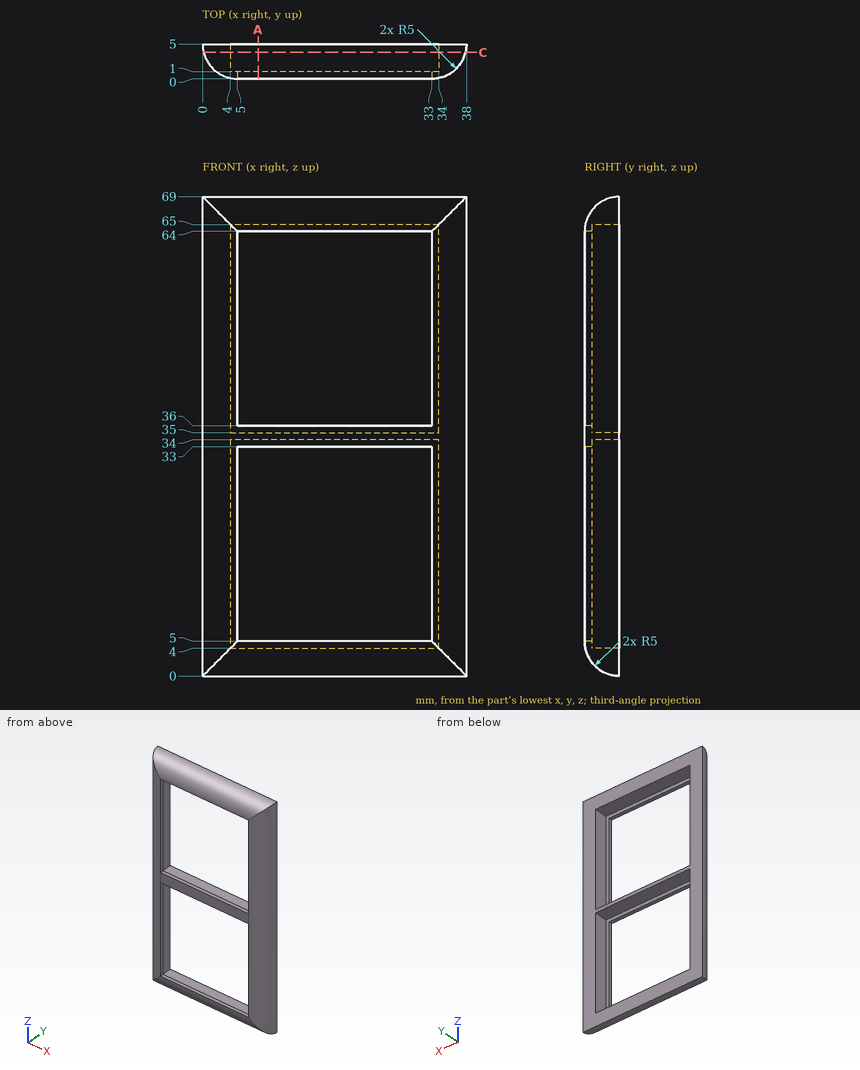
Geometry check sheet. Reference: drawing and pictorial views, mm from the part's lowest x, y, z. Coordinates: 2 decimals unless noted, no trailing zeros. Order: outer loops, then holes, each group sorted by start corner. A loop starts at its lowest first (then second) coordinate and runs counter-clockwise, first axis right, second up.
Item 1: Depth check by flat-ended pin: pin 1 (1.1 mm diameter, centred on y = 0.5, z = 17.5, fed in from -X); pin 2 (1.1 mm diameter, centred on y = 0.5, z = 21, fed in from +X); pin 3 (1.2 mm diameter, centred on y = 3.5, z = 46, fed in from -X). Enter the tip coordinate at first touch or a pass-through.
Item 2: Section check C-C (y = 3.8). Enter the section's corners in (x, z), plus the area to 3 significant figures.
Item 3: Scan lines: line 1 along Z through (x, y) = (8, 4.7); line 2 along X through (y, z) = (4.6, 59.5); line 3 along Z through (x, y) = (25, 1.8). Record each from-to range of solid material in increasing order.
Item 4: Section check A-A (x = 8). Count the separate pieces of the cut face and the enclosed holes in it, plus the area to 3 significant figures.
Check sheet entries:
1. pin 1: stops at x = 1.93
1. pin 2: stops at x = 36.07
1. pin 3: stops at x = 0.08
2. outline: (0.15, 0.15) - (37.85, 0.15) - (37.85, 68.85) - (0.15, 68.85) - close; hole (4, 4) - (34, 4) - (34, 34) - (4, 34) - close; hole (4, 35) - (34, 35) - (34, 65) - (4, 65) - close
2. area: 791 mm2
3. line 1: z = 0.01 to 4, 34 to 35, 65 to 68.99
3. line 2: x = 0.02 to 4, 34 to 37.98
3. line 3: z = 1.16 to 4, 34 to 35, 65 to 67.84
4. separate pieces: 3
4. enclosed holes: 0
4. area: 38.3 mm2
